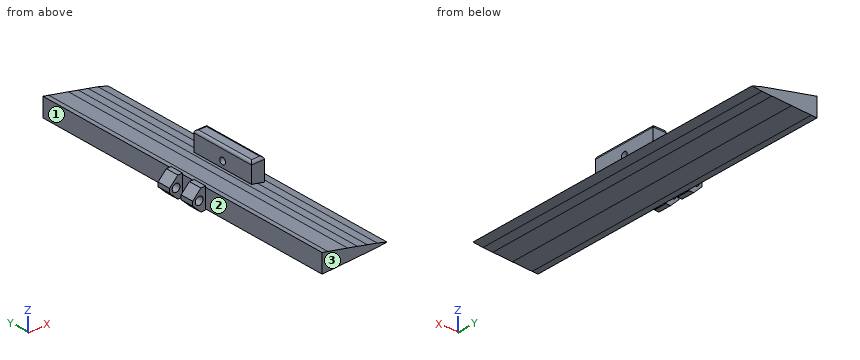
from build123d import *

# Parameters (mm, degrees)
SKETCH023_R  = 1.5
PAD009_DEPTH = 5
SKETCH022_R  = 1.5
PAD012_DEPTH = 5
SKETCH026_W  = 25
SKETCH026_H  = 10
SKETCH026_R  = 1.25
PAD015_DEPTH = 5
FILLET001_R  = 1


with BuildPart() as body015:
    # Sketch023 → Pad009 (new body)
    with BuildSketch(Plane(origin=(0.02, 0, 0), x_dir=(1, 0, 0), z_dir=(0, -1, 0))):
        Polygon((0.683099, -4), (2.5, -4), (2.5, 4), (0.683099, 4), (-2.5, 0.816901), (-2.5, -0.816901), align=None)
        Circle(SKETCH023_R, mode=Mode.SUBTRACT)
    extrude(amount=PAD009_DEPTH)


with BuildPart() as body015_1:
    # Body015 placement: moved
    add(body015.part.moved(Location((362.5, 807.5, 2.5))))


with BuildPart() as body014:
    # Sketch022 → Pad012 (new body)
    with BuildSketch(Plane(origin=(0.02, 0, 0), x_dir=(1, 0, 0), z_dir=(0, -1, 0))):
        Polygon((0.683099, -4), (2.5, -4), (2.5, 4), (0.683099, 4), (-2.5, 0.816901), (-2.5, -0.816901), align=None)
        Circle(SKETCH022_R, mode=Mode.SUBTRACT)
    extrude(amount=PAD012_DEPTH)


with BuildPart() as body014_1:
    # Body014 placement: moved
    add(body014.part.moved(Location((362.5, 817.5, 2.5))))


with BuildPart() as hinge_flap:
    # Sketch026 → Pad015 (new body)
    with BuildSketch(Plane.YZ):
        Rectangle(SKETCH026_W, SKETCH026_H)
        Circle(SKETCH026_R, mode=Mode.SUBTRACT)
    extrude(amount=PAD015_DEPTH)

    # Fillet001
    fillet001_edges = [hinge_flap.edges().sort_by_distance(p)[0] for p in [
        (2.5, 12.5, 5),
        (2.5, -12.5, 5),
        (0, 0, 5),
        (5, 0, 5),
    ]]
    fillet(fillet001_edges, radius=FILLET001_R)


with BuildPart() as hinge_flap_1:
    # Body018 placement: moved
    add(hinge_flap.part.moved(Location((380, 812, 5))))


with BuildPart() as flap:
    # Sketch013 → AdditiveLoft002 section 0
    with BuildSketch(Plane(origin=(10, 873, 0), x_dir=(1, 0, 0), z_dir=(0, -1, 0))):
        Polygon((357.2, 5.557082), (364.8, 3.808816), (368.6, 2.920984), (372.4, 2.02673), (376.2, 1.12822), (380, 0), (376.2, -0.367308), (372.4, -0.506882), (368.6, -0.646418), (364.8, -0.785954), (357.2, -1.065064), (355.003606, -1.145727), (355.003606, 6.050359), align=None)
    # Sketch015 → AdditiveLoft002 section 1
    with BuildSketch(Plane(origin=(10, 752, 0), x_dir=(1, 0, 0), z_dir=(0, -1, 0))):
        Polygon((357.2, 5.557082), (364.8, 3.808816), (368.6, 2.920984), (372.4, 2.02673), (376.2, 1.12822), (380, 0), (376.2, -0.367308), (372.4, -0.506882), (368.6, -0.646418), (364.8, -0.785954), (357.2, -1.065064), (355.003606, -1.145727), (355.003606, 6.050359), align=None)
    loft()

    # Boolean003: union Body015, Body014
    add(body015_1.part)
    add(body014_1.part)

    # Boolean005: union hinge_flap
    add(hinge_flap_1.part)


solid = flap.part
Verification items for the finished model (mm, model axes). Face numbers are marked on the shaded views. A direction names the side the tool comes from. Give positions to 0.01 mm unless a question says otherwise; leave off trailing zeros. Loops run counter-clockwise (first coordinate to the right, second up) from the corner with the lowest first, then second, coordinate; pieces in that order, holes last. Notation, with made-up numbers: (84, -5.75) - (88, -5.75) arc R23 cw to (88, 24.25) - close; hole circle Ø3 at (28, -21.75). An arc over 180 degrees is marked (long way). Write item = value, one per line. Start each with the question number.
Q1. Depth check by flat-ended pin: P1, Ø0.9, axis at x = 364, y = 805.5, coming from the +Z side; P2, Ø2, axis at y = 836.5, z = 4, coming from the -X side; P3, Ø4, axis at x = 371, y = 768.5, coming from the +Z side. Enter the tip coordinate at first touch or a pass-through.
Q2. Cross-section at B-B, the plane x = 373. Enter the section's corners in (y, z).
Q3. Cross-section at A-A, the plane y = 760.5. Enter the section's corners in (x, z).
Q4. Thickness scan on line 1 (Z direction, x = 381.95, y = 812); line 2 (Y direction, x = 364, z = 4); line 3 (Z direction, x = 362.52, y = 806.25). Record the ranges inside material, lowest first.
Q5. Tool access check on the marked faces 1, 2 and 3. Record the directions out of +Z, -Z, +X, -X, +Y, -Y that give a thin tool (end or side, any length) a straight path to the whole face; none if there is none.
Answer key:
q1.P1 = 6.5
q1.P2 = 365
q1.P3 = 5.14
q2.outline = (752, -0.85) - (873, -0.85) - (873, 4.22) - (752, 4.22) - close
q3.outline = (365, -1.15) - (367.2, -1.07) - (374.8, -0.79) - (382.4, -0.51) - (386.2, -0.37) - (390, 0) - (386.2, 1.13) - (382.4, 2.03) - (378.6, 2.92) - (374.8, 3.81) - (367.2, 5.56) - (365, 6.05) - close
q4.line_1 = -0.52 to 3.75, 6.25 to 10
q4.line_2 = 802.5 to 807.5, 812.5 to 817.5
q4.line_3 = -0.82 to 1, 4 to 5.82
q5.face_1 = +Z, -Z, -X, +Y
q5.face_2 = +Z, -Z, -X, -Y
q5.face_3 = +Z, -Z, +X, -X, -Y
